```python
from build123d import *

# Parameters (mm, degrees)
F0_W     = 762
F0_H     = 76.2
F0_R     = 12.7
F1_DEPTH = 6.35
F2_W     = 9.525
F2_H     = 50.8
F3_DEPTH = 6.351
F4_R     = 1.6002


with BuildPart() as f1:
    # F0 (on Front) → F1 (new body)
    with BuildSketch(Plane.XZ):
        with Locations((381, 38.1)):
            Rectangle(F0_W, F0_H)
        with Locations((63.5, 38.1)):
            Circle(F0_R, mode=Mode.SUBTRACT)
        with Locations((190.5, 38.1)):
            Circle(F0_R, mode=Mode.SUBTRACT)
        with Locations((317.5, 38.1)):
            Circle(F0_R, mode=Mode.SUBTRACT)
        with Locations((444.5, 38.1)):
            Circle(F0_R, mode=Mode.SUBTRACT)
        with Locations((571.5, 38.1)):
            Circle(F0_R, mode=Mode.SUBTRACT)
        with Locations((698.5, 38.1)):
            Circle(F0_R, mode=Mode.SUBTRACT)
    extrude(amount=F1_DEPTH)

    # F2 (on face) → F3 (cut, through all)
    with BuildSketch(Plane.XZ.offset(6.35)):
        with Locations((93.4339, 38.1)):
            Rectangle(F2_W, F2_H)
        with Locations((106.1339, 38.1)):
            Rectangle(F2_W, F2_H)
        with Locations((118.8339, 38.1)):
            Rectangle(F2_W, F2_H)
        with Locations((131.5339, 38.1)):
            Rectangle(F2_W, F2_H)
        with Locations((144.2339, 38.1)):
            Rectangle(F2_W, F2_H)
        with Locations((225.4377, 38.1)):
            Rectangle(F2_W, F2_H)
        with Locations((238.1377, 38.1)):
            Rectangle(F2_W, F2_H)
        with Locations((250.8377, 38.1)):
            Rectangle(F2_W, F2_H)
        with Locations((263.5377, 38.1)):
            Rectangle(F2_W, F2_H)
        with Locations((276.2377, 38.1)):
            Rectangle(F2_W, F2_H)
        with Locations((352.4377, 38.1)):
            Rectangle(F2_W, F2_H)
        with Locations((365.1377, 38.1)):
            Rectangle(F2_W, F2_H)
        with Locations((377.8377, 38.1)):
            Rectangle(F2_W, F2_H)
        with Locations((390.5377, 38.1)):
            Rectangle(F2_W, F2_H)
        with Locations((403.2377, 38.1)):
            Rectangle(F2_W, F2_H)
        with Locations((479.4377, 38.1)):
            Rectangle(F2_W, F2_H)
        with Locations((492.1377, 38.1)):
            Rectangle(F2_W, F2_H)
        with Locations((504.8377, 38.1)):
            Rectangle(F2_W, F2_H)
        with Locations((517.5377, 38.1)):
            Rectangle(F2_W, F2_H)
        with Locations((530.2377, 38.1)):
            Rectangle(F2_W, F2_H)
        with Locations((606.4377, 38.1)):
            Rectangle(F2_W, F2_H)
        with Locations((619.1377, 38.1)):
            Rectangle(F2_W, F2_H)
        with Locations((631.8377, 38.1)):
            Rectangle(F2_W, F2_H)
        with Locations((644.5377, 38.1)):
            Rectangle(F2_W, F2_H)
        with Locations((657.2377, 38.1)):
            Rectangle(F2_W, F2_H)
    extrude(amount=-F3_DEPTH, mode=Mode.SUBTRACT)

    # F4
    f4_edges = [f1.edges().sort_by_distance(p)[0] for p in [
        (381, -6.35, 76.2),
        (381, 0, 76.2),
        (0, -6.35, 38.1),
        (0, 0, 38.1),
        (762, -3.175, 76.2),
        (0, -3.175, 76.2),
        (0, -3.175, 0),
        (381, -6.35, 0),
        (381, 0, 0),
        (762, -3.175, 0),
        (762, -6.35, 38.1),
    ]]
    fillet(f4_edges, radius=F4_R)


solid = f1.part
```
Geometry: final body of the model. Coordinates: model frame, mm. Coordinates: 2 decimals unless noted, no trailing zeros. Order: outer loops, then holes, each group sorted by start corner. A loop starts at its lowest first (then second) coordinate and runs counter-clockwise, first axis right, second up. Notation, with made-up numbers: M 68,49.5 L 74,49.5 A8 cw 74,54.5 Z; hole C 76.5,45.25 d4. An arc over 180 degrees is marked long. Answer in a Markdown table with one row per item. Add a question column.
Q1. Section query B-B on z = 38.1. Count the separate pieces of the cut face and the enclosed holes in it, and give its area (3 significant figures).
Q2. Section query C-C on x = 69. Return the cut outline in (y, z).
Q3. Section query A-A on x = 571.5. Return the cut outline in (y, z), and give its area (3 significant figures).
Q4. Mould query, pull axis X, two halves, no side actions, for faces 1 (the flat face through (376, -6.35, 6)), 2 (the cylindrical face through (558.812, -3.131, 38.658)). Classes: released by +X, released by -X, zero draft, split by the parting line, or undercut.
Q5. Line query: L1, parallel to Z at x = 698.5, y = -2; L2, parallel to Z at x = 576, y = -5. Output: solid intervals per line, ascending.
Completed:
| question | item | result |
|---|---|---|
| 1 | separate pieces | 32 |
| 1 | enclosed holes | 0 |
| 1 | area | 2,360 mm2 |
| 2 | outline | M -6.35,1.6 A1.6 ccw -4.75,0 L -1.6,0 A1.6 ccw 0,1.6 L 0,26.65 L -6.35,26.65 Z; M -6.35,49.55 L 0,49.55 L 0,74.6 A1.6 ccw -1.6,76.2 L -4.75,76.2 A1.6 ccw -6.35,74.6 Z |
| 3 | outline | M -6.35,1.6 A1.6 ccw -4.75,0 L -1.6,0 A1.6 ccw 0,1.6 L 0,25.4 L -6.35,25.4 Z; M -6.35,50.8 L 0,50.8 L 0,74.6 A1.6 ccw -1.6,76.2 L -4.75,76.2 A1.6 ccw -6.35,74.6 Z |
| 3 | area | 320 mm2 |
| 4 | face 1 | zero draft |
| 4 | face 2 | undercut |
| 5 | L1 | z = 0 to 25.4, 50.8 to 76.2 |
| 5 | L2 | z = 0.02 to 26.22, 49.98 to 76.18 |
